```python
from build123d import *

# Parameters (mm, degrees)
SKETCH1_W           = 150
SKETCH1_H           = 60
BOSS_EXTRUDE1_DEPTH = 90
SKETCH2_W           = 144.92
SKETCH2_H           = 60
CUT_EXTRUDE1_DEPTH  = 85
SKETCH6_R           = 2.499995
SKETCH6_R_2         = 1.25
BOSS_EXTRUDE2_DEPTH = 2
BOSS_EXTRUDE3_DEPTH = 2
SKETCH8_W           = 8.5
SKETCH8_H           = 4
CUT_EXTRUDE4_DEPTH  = 2.54
SKETCH12_W          = 80
SKETCH12_H          = 30
BOSS_EXTRUDE5_DEPTH = 10
SKETCH13_W          = 75
SKETCH13_H          = 25
CUT_EXTRUDE6_DEPTH  = 10
SKETCH16_W          = 1.27
SKETCH16_H          = 2.54
CUT_EXTRUDE7_DEPTH  = 85


with BuildPart() as part:
    # Sketch1 → Boss-Extrude1 (new body)
    with BuildSketch(Plane(origin=(0, 0, 0), x_dir=(1, 0, 0), z_dir=(0, 1, 0))):
        Rectangle(SKETCH1_W, SKETCH1_H)
    extrude(amount=BOSS_EXTRUDE1_DEPTH)

    # Sketch2 → Cut-Extrude1 (cut)
    with BuildSketch(Plane(origin=(0, 90, 0), x_dir=(1, 0, 0), z_dir=(0, 1, 0))):
        with Locations((0, -2.54)):
            Rectangle(SKETCH2_W, SKETCH2_H)
    extrude(amount=-CUT_EXTRUDE1_DEPTH, mode=Mode.SUBTRACT)

    # Sketch6 → Boss-Extrude2 (add)
    # profile 1 of 4: a face of its own
    with BuildSketch(Plane.XY.offset(-27.46)):
        with Locations(Location((-2.46, 39.829239544, 0), (0, 0, 180))):
            Circle(SKETCH6_R)
        with Locations((-2.46, 39.829239544)):
            Circle(SKETCH6_R_2, mode=Mode.SUBTRACT)
    # profile 2 of 4: a face of its own
    with BuildSketch(Plane.XY.offset(-27.46)):
        with Locations(Location((55.54, 39.829239544, 0), (0, 0, 180))):
            Circle(SKETCH6_R)
        with Locations((55.54, 39.829239544)):
            Circle(SKETCH6_R_2, mode=Mode.SUBTRACT)
    # profile 3 of 4: a face of its own
    with BuildSketch(Plane.XY.offset(-27.46)):
        with Locations(Location((55.54, 16.829239544, 0), (0, 0, 180))):
            Circle(SKETCH6_R)
        with Locations((55.54, 16.829239544)):
            Circle(SKETCH6_R_2, mode=Mode.SUBTRACT)
    # profile 4 of 4: a face of its own
    with BuildSketch(Plane.XY.offset(-27.46)):
        with Locations(Location((-2.46, 16.829239544, 0), (0, 0, 180))):
            Circle(SKETCH6_R)
        with Locations((-2.46, 16.829239544)):
            Circle(SKETCH6_R_2, mode=Mode.SUBTRACT)
    extrude(amount=BOSS_EXTRUDE2_DEPTH)

    # Sketch7 → Boss-Extrude3 (add)
    with BuildSketch(Plane.XY.offset(-27.46)):
        Polygon((-38.17, 24.030063331), (-38.17, 22.030063331), (-33.17, 22.030063331), (-33.17, 27.030063331), (-35.17, 27.030063331), (-35.17, 24.030063331), align=None)
    extrude(amount=BOSS_EXTRUDE3_DEPTH)

    # Sketch8 → Cut-Extrude4 (cut)
    with BuildSketch(Plane.ZY.offset(75)):
        with Locations((-1, 11.52476666)):
            Rectangle(SKETCH8_W, SKETCH8_H)
    extrude(amount=-CUT_EXTRUDE4_DEPTH, mode=Mode.SUBTRACT)

    # Sketch12 → Boss-Extrude5 (add)
    with BuildSketch(Plane(origin=(0, 5, 0), x_dir=(1, 0, 0), z_dir=(0, 1, 0))):
        with Locations((0.430037325, 0.273645115)):
            Rectangle(SKETCH12_W, SKETCH12_H)
    extrude(amount=BOSS_EXTRUDE5_DEPTH)

    # Sketch13 → Cut-Extrude6 (cut)
    with BuildSketch(Plane(origin=(0, 15, 0), x_dir=(1, 0, 0), z_dir=(0, 1, 0))):
        with Locations((0.430037325, 0.273645115)):
            Rectangle(SKETCH13_W, SKETCH13_H)
    extrude(amount=-CUT_EXTRUDE6_DEPTH, mode=Mode.SUBTRACT)

    # Sketch16 → Cut-Extrude7 (cut)
    with BuildSketch(Plane(origin=(0, 90, 0), x_dir=(1, 0, 0), z_dir=(0, 1, 0))):
        with Locations((-73.095, -27.46)):
            Rectangle(SKETCH16_W, SKETCH16_H)
        with Locations((73.095, -27.46)):
            Rectangle(SKETCH16_W, SKETCH16_H)
    extrude(amount=-CUT_EXTRUDE7_DEPTH, mode=Mode.SUBTRACT)


solid = part.part
```
Verification items for the finished model (mm, model axes). A direction names the side the tool comes from. Coordinates: 2 decimals unless noted, no trailing zeros. Loops run counter-clockwise (first coordinate to the right, second up) from the corner with the lowest first, then second, coordinate; pieces in that order, holes last. Notation, with made-up numbers: (14, 15.5) - (39, 15.5) arc R27 cw to (39, 42.5) - close; hole circle Ø5 at (21, 84.5). An arc over 180 degrees is marked (long way). Return JSON: item names as keys, results as strings.
1. Tool access check on faces 5 (the cylindrical face through (-2.13, 37.35, -26.47)), 6 (the flat face through (57, 17, -25.46)), 7 (the flat face through (0, 10, -15.274)). Record the directions out of +Z, -Z, +X, -X, +Y, -Y that give a thin tool (end or side, any length) a straight path to the whole face; none if there is none.
Established:
{"face 5": "+Z", "face 6": "+Z, +Y", "face 7": "+Y"}
2. Mould release check, pull along Y, two halves, no side actions. Record for faces 1 (the flat face through (-1, 0, 0)), 2 (the flat face through (0, 5, 0)), 3 (the cylindrical face through (58.038, 16.719, -26.474)), 4 (the flat face through (-22.6, 4.8, 30)): +Y half, -Y half, draft (parallel to the pull), parting line (faces both ways), or undercut.
Established:
{"face 1": "-Y half", "face 2": "+Y half", "face 3": "undercut", "face 4": "draft"}
3. Thickness scan on L1, parallel to X at y = 66, z = -11.5; L2, parallel to Y at x = -2, z = -26; L3, parallel to X at y = 14.5, z = -9.5. Record the ranges inside material, lowest first.
Established:
{"L1": "x = -75 to -72.46, 72.46 to 75", "L2": "y = 0 to 5, 14.37 to 15.67, 17.99 to 19.29, 37.37 to 38.67, 40.99 to 42.29", "L3": "x = -75 to -72.46, -39.57 to -37.07, 37.93 to 40.43, 72.46 to 75"}
4. Section check C-C, the plane z = -18. Record the boundary of the cut face in (x, y).
Established:
{"outline": "(-75, 0) - (75, 0) - (75, 90) - (72.46, 90) - (72.46, 5) - (-72.46, 5) - (-72.46, 90) - (-75, 90) - close"}
5. Section check B-B, the plane y = 29. Record the boundary of the cut face in (x, z), then the cut area to 3 significant figures.
Established:
{"outline": "(-75, -30) - (75, -30) - (75, 30) - (72.46, 30) - (72.46, 28.73) - (73.73, 28.73) - (73.73, 26.19) - (72.46, 26.19) - (72.46, -27.46) - (-72.46, -27.46) - (-72.46, 26.19) - (-73.73, 26.19) - (-73.73, 28.73) - (-72.46, 28.73) - (-72.46, 30) - (-75, 30) - close", "area": "666 mm2"}
6. Section check D-D, the plane x = 47. Record the boundary of the cut face in (y, z).
Established:
{"outline": "(0, -30) - (90, -30) - (90, -27.46) - (5, -27.46) - (5, 30) - (0, 30) - close"}
7. Go/stop test with flat-tipped pins: pin 1 (2 mm diameter, centred on x = 55.54, y = 16.83, fed in from +Z); pin 2 (3 mm diameter, centred on x = -2.46, y = 39.83, fed in from +Z). Record where each tip stops, or that it passes through.
Established:
{"pin 1": "stops at z = -27.46", "pin 2": "stops at z = -25.46"}
8. Section check A-A, the plane z = 0. Record the boundary of the cut face in (x, y), then the cut area to 3 significant figures.
Established:
{"outline": "(-75, 0) - (75, 0) - (75, 90) - (72.46, 90) - (72.46, 5) - (40.43, 5) - (40.43, 15) - (37.93, 15) - (37.93, 5) - (-37.07, 5) - (-37.07, 15) - (-39.57, 15) - (-39.57, 5) - (-72.46, 5) - (-72.46, 9.52) - (-75, 9.52) - close; (-75, 13.52) - (-72.46, 13.52) - (-72.46, 90) - (-75, 90) - close", "area": "1,220 mm2"}
